from build123d import *

# Parameters (mm, degrees)
SKETCH1_W                          = 180
SKETCH1_H                          = 120
BOSS_EXTRUDE1_DEPTH                = 20
CUT_EXTRUDE1_DEPTH                 = 15
SKETCH3_W                          = 25
SKETCH3_H                          = 34.37
CUT_EXTRUDE2_DEPTH                 = 15
MIRROR2_COPY_1_SKETCH_W            = 25
MIRROR2_COPY_1_SKETCH_H            = 34.37
MIRROR2_COPY_1_DEPTH               = 15
SKETCH4_W                          = 96.808518295
SKETCH4_H                          = 75.84152956
CUT_EXTRUDE4_DEPTH                 = 10
SKETCH6_R                          = 1.750328968
SKETCH6_R_2                        = 1.75
BOSS_EXTRUDE2_DEPTH                = 2.5
F_2_0_2_DIAMETER_HOLE1_D           = 2
F_2_0_2_DIAMETER_HOLE1_DEPTH       = 2
F_2_0_2_DIAMETER_HOLE1_CSINK_D     = 2.05
F_2_0_2_DIAMETER_HOLE1_CSINK_ANGLE = 92
F_2_0_2_DIAMETER_HOLE1_TIP         = 0.600860619
CUT_EXTRUDE5_DEPTH                 = 10
SKETCH23_R                         = 2
BOSS_EXTRUDE3_DEPTH                = 5
SKETCH25_W                         = 5.325181223
SKETCH25_H                         = 5.082469794
SKETCH25_H_2                       = 4.706000646
CUT_EXTRUDE10_DEPTH                = 4
CUT_EXTRUDE11_DEPTH                = 5
SKETCH28_W                         = 81.316631719
SKETCH28_H                         = 14.691658707
CUT_EXTRUDE12_DEPTH                = 10
SKETCH29_W                         = 55.195697226
SKETCH29_H                         = 2.199341939
CUT_EXTRUDE13_DEPTH                = 5
SKETCH30_W                         = 23.172037828
SKETCH30_H                         = 3.131356463
SKETCH30_H_2                       = 2.952421808
SKETCH30_W_2                       = 20.586646559
CUT_EXTRUDE15_DEPTH                = 110.201648339
SKETCH31_W                         = 55.195697226
SKETCH31_H                         = 0.376469148
CUT_EXTRUDE16_DEPTH                = 5
SKETCH32_W                         = 20
SKETCH32_H                         = 10
CUT_EXTRUDE17_DEPTH                = 15
CUT_EXTRUDE18_DEPTH                = 5


with BuildPart() as part:
    # Sketch1 → Boss-Extrude1 (new body)
    with BuildSketch(Plane(origin=(0, 0, 0), x_dir=(1, 0, 0), z_dir=(0, 1, 0))):
        Rectangle(SKETCH1_W, SKETCH1_H)
    extrude(amount=BOSS_EXTRUDE1_DEPTH)

    # Sketch2 → Cut-Extrude1 (cut)
    with BuildSketch(Plane(origin=(0, 20, 0), x_dir=(1, 0, 0), z_dir=(0, 1, 0))):
        Polygon((90, 0), (90, 27.5), (20, 27.5), (20, -27.5), (90, -27.5), align=None)
    extrude(amount=-CUT_EXTRUDE1_DEPTH, mode=Mode.SUBTRACT)

    # Sketch3 → Cut-Extrude2 (cut)
    with BuildSketch(Plane(origin=(0, 20, 0), x_dir=(1, 0, 0), z_dir=(0, 1, 0))):
        with Locations((55.95586419, -60)):
            Rectangle(SKETCH3_W, SKETCH3_H)
    cut_extrude2 = extrude(amount=-CUT_EXTRUDE2_DEPTH, mode=Mode.SUBTRACT)

    # Mirror1: Cut-Extrude2 across plane
    add(cut_extrude2.mirror(Plane(origin=(0, 0, 0), x_dir=(0, 0, 1), z_dir=(1, 0, 0))), mode=Mode.SUBTRACT)

    # Mirror2: Cut-Extrude2 across plane
    add(cut_extrude2.mirror(Plane.XY), mode=Mode.SUBTRACT)

    # Mirror2 copy 1 sketch → Mirror2 copy 1 (cut)
    with BuildSketch(Plane(origin=(0, 20, 0), x_dir=(-1, 0, 0), z_dir=(0, 1, 0))):
        with Locations((55.95586419, -60)):
            Rectangle(MIRROR2_COPY_1_SKETCH_W, MIRROR2_COPY_1_SKETCH_H)
    extrude(amount=-MIRROR2_COPY_1_DEPTH, mode=Mode.SUBTRACT)

    # Sketch4 → Cut-Extrude4 (cut)
    with BuildSketch(Plane(origin=(0, 20, 0), x_dir=(1, 0, 0), z_dir=(0, 1, 0))):
        with Locations((-34.664426112, 0.188234574)):
            Rectangle(SKETCH4_W, SKETCH4_H)
    extrude(amount=-CUT_EXTRUDE4_DEPTH, mode=Mode.SUBTRACT)

    # Sketch6 → Boss-Extrude2 (add)
    with BuildSketch(Plane(origin=(0, 5, 0), x_dir=(1, 0, 0), z_dir=(0, 1, 0))):
        with Locations(Location((23.740233284, 19.759861377, 0), (0, 0, 270))):
            Circle(SKETCH6_R)
        with Locations(Location((23.740233284, -8.257995296, 0), (0, 0, 270))):
            Circle(SKETCH6_R_2)
        with Locations(Location((74.958841447, -23.692393533, 0), (0, 0, 270))):
            Circle(SKETCH6_R_2)
    extrude(amount=BOSS_EXTRUDE2_DEPTH)

    # Ø2.0 (2) Diameter Hole1
    with Locations(Plane(origin=(23.740233284, 7.5, -19.759861377), x_dir=(0, 0, 1), z_dir=(0, 1, 0))):
        with Locations((0, 0), (28.017856673, 0), (43.45225491, 51.218608163)):
            CounterSinkHole(F_2_0_2_DIAMETER_HOLE1_D / 2, F_2_0_2_DIAMETER_HOLE1_CSINK_D / 2, depth=F_2_0_2_DIAMETER_HOLE1_DEPTH, counter_sink_angle=F_2_0_2_DIAMETER_HOLE1_CSINK_ANGLE)
            with Locations((0, 0, -(F_2_0_2_DIAMETER_HOLE1_DEPTH + F_2_0_2_DIAMETER_HOLE1_TIP / 2))):  # 118° drill point
                Cone(0, F_2_0_2_DIAMETER_HOLE1_D / 2, F_2_0_2_DIAMETER_HOLE1_TIP, mode=Mode.SUBTRACT)

    # Sketch19 → Cut-Extrude5 (cut)
    with BuildSketch(Plane(origin=(20, 0, 0), x_dir=(0, 0, -1), z_dir=(1, 0, 0))):
        with BuildLine():
            Line((-17.205162996, 24.206637085), (16.076682843, 24.206637085))
            ThreePointArc((16.076682843, 24.206637085), (20.283319928, 20), (16.076682843, 15.793362915))
            Line((16.076682843, 15.793362915), (-17.205162996, 15.793362915))
            ThreePointArc((-17.205162996, 15.793362915), (-21.411800081, 20), (-17.205162996, 24.206637085))
        make_face()
    extrude(amount=-CUT_EXTRUDE5_DEPTH, mode=Mode.SUBTRACT)

    # Sketch23 → Boss-Extrude3 (add)
    with BuildSketch(Plane(origin=(0, 20, 0), x_dir=(1, 0, 0), z_dir=(0, 1, 0))):
        with Locations(Location((-85, 55, 0), (0, 0, 90))):
            Circle(SKETCH23_R)
        with Locations(Location((-85, -55, 0), (0, 0, 90))):
            Circle(SKETCH23_R)
    boss_extrude3 = extrude(amount=BOSS_EXTRUDE3_DEPTH)

    # Mirror3: Boss-Extrude3 across plane
    add(boss_extrude3.mirror(Plane(origin=(0, 0, 0), x_dir=(0, 0, 1), z_dir=(1, 0, 0))))

    # Sketch25 → Cut-Extrude10 (cut)
    with BuildSketch(Plane(origin=(0, 20, 0), x_dir=(1, 0, 0), z_dir=(0, 1, 0))):
        with Locations((-57.266281273, -40.273765103)):
            Rectangle(SKETCH25_W, SKETCH25_H)
        with Locations((-57.266281273, 40.461999677)):
            Rectangle(SKETCH25_W, SKETCH25_H_2)
    extrude(amount=-CUT_EXTRUDE10_DEPTH, mode=Mode.SUBTRACT)

    # Sketch27 → Cut-Extrude11 (cut)
    with BuildSketch(Plane(origin=(0, 20, 0), x_dir=(1, 0, 0), z_dir=(0, 1, 0))):
        with BuildLine():
            Line((53.518871282, -42.815), (53.518871282, -34.725256946))
            ThreePointArc((53.518871282, -34.725256946), (55.95586419, -32.288264038), (58.392857098, -34.725256946))
            Line((58.392857098, -34.725256946), (58.392857098, -42.815))
            ThreePointArc((58.392857098, -42.815), (55.95586419, -45.251992908), (53.518871282, -42.815))
        make_face()
        with BuildLine():
            Line((55.95586419, -36.875864951), (13.739833036, -36.875864951))
            ThreePointArc((13.739833036, -36.875864951), (11.589225031, -34.725256946), (13.739833036, -32.574648942))
            Line((13.739833036, -32.574648942), (55.95586419, -32.574648942))
            ThreePointArc((55.95586419, -32.574648942), (58.106472195, -34.725256946), (55.95586419, -36.875864951))
        make_face()
    cut_extrude11 = extrude(amount=-CUT_EXTRUDE11_DEPTH, mode=Mode.SUBTRACT)

    # Mirror4: Cut-Extrude11 across plane
    add(cut_extrude11.mirror(Plane.XY), mode=Mode.SUBTRACT)

    # Sketch28 → Cut-Extrude12 (cut)
    with BuildSketch(Plane(origin=(0, 20, 0), x_dir=(1, 0, 0), z_dir=(0, 1, 0))):
        with Locations((-0.79754833, 47.654170647)):
            Rectangle(SKETCH28_W, SKETCH28_H)
    cut_extrude12 = extrude(amount=-CUT_EXTRUDE12_DEPTH, mode=Mode.SUBTRACT)

    # Sketch29 → Cut-Extrude13 (cut)
    with BuildSketch(Plane(origin=(0, 20, 0), x_dir=(1, 0, 0), z_dir=(0, 1, 0))):
        with Locations((-13.858015577, 39.208670324)):
            Rectangle(SKETCH29_W, SKETCH29_H)
    cut_extrude13 = extrude(amount=-CUT_EXTRUDE13_DEPTH, mode=Mode.SUBTRACT)

    # Sketch30 → Cut-Extrude15 (cut, through all)
    with BuildSketch(Plane(origin=(0, 10, 0), x_dir=(1, 0, 0), z_dir=(0, 1, 0))):
        with Locations((19.694260821, 52.169495653)):
            Rectangle(SKETCH30_W, SKETCH30_H)
        with Locations((19.694260821, 44.206903503)):
            Rectangle(SKETCH30_W, SKETCH30_H_2)
        with Locations((-23.35450663, 52.169495653)):
            Rectangle(SKETCH30_W_2, SKETCH30_H)
        with Locations((-23.35450663, 44.206903503)):
            Rectangle(SKETCH30_W_2, SKETCH30_H_2)
    cut_extrude15 = extrude(amount=-CUT_EXTRUDE15_DEPTH, mode=Mode.SUBTRACT)

    # Mirror5: Cut-Extrude12, Cut-Extrude13, Cut-Extrude15 across plane
    add(cut_extrude12.mirror(Plane.XY), mode=Mode.SUBTRACT)
    add(cut_extrude13.mirror(Plane.XY), mode=Mode.SUBTRACT)
    add(cut_extrude15.mirror(Plane.XY), mode=Mode.SUBTRACT)

    # Sketch31 → Cut-Extrude16 (cut)
    with BuildSketch(Plane(origin=(0, 20, 0), x_dir=(1, 0, 0), z_dir=(0, 1, 0))):
        with Locations((-13.858015577, -37.92076478)):
            Rectangle(SKETCH31_W, SKETCH31_H)
    extrude(amount=-CUT_EXTRUDE16_DEPTH, mode=Mode.SUBTRACT)

    # Sketch32 → Cut-Extrude17 (cut)
    with BuildSketch(Plane(origin=(90, 0, 0), x_dir=(0, 0, -1), z_dir=(1, 0, 0))):
        with Locations((-41.109013554, 15)):
            Rectangle(SKETCH32_W, SKETCH32_H)
    extrude(amount=-CUT_EXTRUDE17_DEPTH, mode=Mode.SUBTRACT)

    # Sketch33 → Cut-Extrude18 (cut)
    with BuildSketch(Plane(origin=(0, 20, 0), x_dir=(1, 0, 0), z_dir=(0, 1, 0))):
        with BuildLine():
            Line((55.95586419, -32.253444684), (75, -32.253444684))
            ThreePointArc((75, -32.253444684), (77.471812262, -34.725256946), (75, -37.197069209))
            Line((75, -37.197069209), (55.95586419, -37.197069209))
            ThreePointArc((55.95586419, -37.197069209), (53.484051928, -34.725256946), (55.95586419, -32.253444684))
        make_face()
    extrude(amount=-CUT_EXTRUDE18_DEPTH, mode=Mode.SUBTRACT)


solid = part.part
Geometry: final body of the model. Coordinates: model frame, mm. A direction names the side the tool comes from. Give positions to 0.01 mm unless a question says otherwise; leave off trailing zeros. Order: outer loops, then holes, each group sorted by start corner. A loop starts at its lowest first (then second) coordinate and runs counter-clockwise, first axis right, second up. Notation, with made-up numbers: (-27.75, -13) -> (31.25, -13) arc R23 ccw to (31.25, -3) -> close; hole circle Ø7 at (66, -1.5). An arc over 180 degrees is marked (long way). Answer as a JSON object with one key per item and string values.
Q1. Section B-B (z = 0.5). Output: boundary loops of the cut face in (x, y), plus the area to 3 significant figures.
Entries:
{"outline": "(-90, 0) -> (90, 0) -> (90, 5) -> (20, 5) -> (20, 15.79) -> (13.74, 15.79) -> (13.74, 10) -> (-83.07, 10) -> (-83.07, 20) -> (-90, 20) -> close", "area": "1,560 mm^2"}
Q2. Section A-A (x = -22). State how many separate pieces and enclosed holes the cut face has, plus the area to 3 significant figures.
Entries:
{"separate pieces": "5", "enclosed holes": "0", "area": "1,200 mm^2"}
Q3. Access query for faces 1 (the flat face through (20, 5, 53.735)), 2 (the flat face through (58.393, 18, 40)), 3 (the flat face through (83, 10, 41)). Directions: +Z, -Z, +X, -X, +Y, -Y. A direction counts if a zero-diameter tool reaches every point of the face in a straight line with its end or side. Return the directions, or none.
Entries:
{"face 1": "+Y, -Y", "face 2": "+Z, +Y", "face 3": "+X, +Y"}
Q4. First-contact query: pin 1 (2 mm diameter, centred on y = 7, z = -4, fed in from +X); pin 2 (12 mm diameter, centred on x = 55.5, y = 15.5, fed in from +Z) (3 decimals); pin 3 (11.5 mm diameter, centred on x = 44.5, z = 36, fed in from +Y). Flat tips, straight axial feed; report the tip coordinate or a pass-through.
Entries:
{"pin 1": "stops at x = 20", "pin 2": "stops at z = 42.815", "pin 3": "stops at y = 20"}
Q5. Section C-C (x = 2.5). Output: boundary loops of the cut face in (y, z), plus the area to 3 significant figures.
Entries:
{"outline": "(0, -60) -> (20, -60) -> (20, -55) -> (10, -55) -> (10, -40.31) -> (15, -40.31) -> (15, -38.11) -> (10, -38.11) -> (10, 37.73) -> (15, 37.73) -> (15, 40.31) -> (10, 40.31) -> (10, 55) -> (20, 55) -> (20, 60) -> (0, 60) -> close", "area": "1,320 mm^2"}
Q6. Section D-D (y = 23.25). Output: boundary loops of the cut face in (x, z).
Entries:
{"outline": "circle Ø4 at (-85, -55); circle Ø4 at (-85, 55); circle Ø4 at (85, -55); circle Ø4 at (85, 55)"}
Q7. Material intervals for probe 1 along Z at (x, y) = (-33, 8.5); probe 2 along X at (y, z) = (1.5, -45); probe 3 along X at (y, z) = (11, 2.5), sorted ascending.
Entries:
{"probe 1": "z = -60 to -53.74, -50.6 to -45.68, -42.73 to 42.73, 45.68 to 50.6, 53.74 to 60", "probe 2": "x = -90 to -33.65, -13.06 to 8.11, 31.28 to 90", "probe 3": "x = -90 to -83.07, 13.74 to 20"}
Q8. Draft query along Z for faces 4 (the flat face through (-56, 5, -51)), 5 (the flat face through (17, 15.793, 0)), 6 (the flat face through (-1, 10, 60)). Return one class per face: released by +Z, released by -Z, zero draft, split by the parting line, or undercut.
Entries:
{"face 4": "zero draft", "face 5": "undercut", "face 6": "released by +Z"}
